Design review of the part built by this model. Coordinates are the model's own, in mm. Face numbers are marked on the shaded views. A direction names the side the tool comes from. Give positions to 0.01 mm unless a question says otherwise; leave off trailing zeros. Write each loop counter-clockwise with the first axis right and the second up, starting at its lowest first coordinate (ties: lowest second). Pieces come first, ordered by that corner, then holes. Notation, with made-up numbers: (-30, -37) -> (-11, -37) arc R3 cw to (-11, -33) -> close; hole circle Ø8 at (38.5, 11.5). An arc over 180 degrees is marked (long way). Write each question's results on one line, items separated by ' | '. Start each with the question number.
(1) Take a section at C-C (x = 117). State the section outline as (y, z) points.
(2) Take a section at D-D (x = 39). State the section outline as (y, z) points.
(3) For the marked faces 1 and 2, list the 3-axis set-ups (+Z, -Z, +X, -X, +Y, -Y) from which the entire face can be reached by the end or side of a thin tool; tool diameter is ignored.
(4) Take a section at A-A (x = -63). State the section outline as (y, z) points.
(5) Clearance check with flat-ended pins moving along their axes: pin 1 (5 mm diameter, centred on x = 9, y = 28.5, fed in from -Z); pin 2 (10 mm diameter, centred on y = 8.5, z = -33, fed in from +X); pin 3 (1.5 mm diameter, centred on y = 30, z = -1, fed in from +X); pin 4 (9 mm diameter, centred on x = 20.99, z = -20.99, fed in from +Y). State where each tip first meets the part, or that it passes through.
(6) Take a section at B-B (y = 2.5). Count the separate pieces of the cut face and the enclosed holes in it, plus the area to 3 significant figures.
(7) Mouldability with a two-part tool opening along Z and no side actions: class the marked faces 3, 4 and 5 as released by +Z, released by -Z, zero draft, split by the parting line, or undercut.
(8) To check wall thickness, follow probe 1 along Z at (x, y) = (-65, 11); probe 2 along Z at (x, y) = (-28, 6); probe 3 along Z at (x, y) = (16.5, 32). State the ranges of each line that lie inside material, in increasing order.
from build123d import *

# Parameters (mm, degrees)
BOSS_EXTRUDE3_DEPTH = 35
SKETCH1_8_R         = 4.99771167
SKETCH1_8_R_2       = 3.998169336
BOSS_EXTRUDE4_DEPTH = 5
CUT_EXTRUDE1_DEPTH  = 10
BOSS_EXTRUDE5_START = -3
SKETCH22_R          = 3
BOSS_EXTRUDE5_DEPTH = 3
SKETCH2_R           = 12
SKETCH2_R_2         = 9.5
BOSS_EXTRUDE6_DEPTH = 29
SKETCH23_R          = 3
SKETCH23_R_2        = 2.999999999
BOSS_EXTRUDE7_DEPTH = 4
SKETCH11_R          = 1.5
SKETCH11_R_2        = 11.25
CUT_EXTRUDE2_DEPTH  = 20
SKETCH24_R          = 4
SKETCH24_R_2        = 2.5
SKETCH24_R_3        = 3.5
SKETCH24_R_4        = 2.500018474
BOSS_EXTRUDE8_DEPTH = 30


with BuildPart() as part:
    # Sketch1 → Boss-Extrude3 (new body)
    with BuildSketch(Plane(origin=(0, 0, 0), x_dir=(1, 0, 0), z_dir=(0, 1, 0))):
        with BuildLine():
            Line((-86.695031893, 25.988113322), (-86.695031893, -25.991886678))
            Line((-86.695031893, -25.991886678), (-39.189227367, -25.991886678))
            ThreePointArc((-39.189227367, -25.991886678), (-7.506053104, -46.403541136), (28.985180603, -36.977564703))
            Line((28.985180603, -36.977564703), (84.985180603, -36.999994064))
            ThreePointArc((84.985180603, -36.999994064), (122.000000001, 2.968e-06), (84.985180603, 37))
            Line((84.985180603, 37), (28.985180603, 36.977570638))
            ThreePointArc((28.985180603, 36.977570638), (-7.510107434, 46.404944207), (-39.195031893, 25.988113322))
            Line((-39.195031893, 25.988113322), (-86.695031893, 25.988113322))
        make_face()
        with BuildLine():
            Line((-82.377665867, 22.997385422), (-82.377665867, -22.999994064))
            Line((-82.377665867, -22.999994064), (-37.526858967, -22.999994064))
            ThreePointArc((-37.526858967, -22.999994064), (-7.29337461, -43.394145047), (27.938898317, -33.977568435))
            Line((27.938898317, -33.977568435), (84.985180603, -34.00091317))
            ThreePointArc((84.985180603, -34.00091317), (119.000007777, -2.847e-06), (84.985180603, 34.000907476))
            Line((84.985180603, 34.000907476), (27.945855319, 33.977565588))
            ThreePointArc((27.945855319, 33.977565588), (-7.280719209, 43.388716375), (-37.507775535, 22.997385422))
            Line((-37.507775535, 22.997385422), (-82.377665867, 22.997385422))
        make_face(mode=Mode.SUBTRACT)
    extrude(amount=BOSS_EXTRUDE3_DEPTH)

    # Sketch22 → Boss-Extrude5 (add)
    with BuildSketch(Plane(origin=(0, 35, 0), x_dir=(1, 0, 0), z_dir=(0, 1, 0)).offset(BOSS_EXTRUDE5_START)):
        with BuildLine():
            ThreePointArc((126, -4), (130, 0), (126, 4))
            Line((126, 4), (121.783148639, 4))
            ThreePointArc((121.783148639, 4), (122.000000001, -1.7e-08), (121.783147994, -4))
            Line((121.783147994, -4), (126, -4))
        make_face()
        with Locations(Location((126, 0, 0), (0, 0, 270))):
            Circle(SKETCH22_R, mode=Mode.SUBTRACT)
    extrude(amount=BOSS_EXTRUDE5_DEPTH)


with BuildPart() as body_2:
    # Sketch1_8 → Boss-Extrude4 (new body)
    with BuildSketch(Plane(origin=(0, 0, 0), x_dir=(1, 0, 0), z_dir=(0, 1, 0))):
        with BuildLine():
            Line((-82.377665867, 22.997385422), (-82.377665867, -22.999994064))
            Line((-82.377665867, -22.999994064), (-37.526858967, -22.999994064))
            ThreePointArc((-37.526858967, -22.999994064), (-7.29337461, -43.394145047), (27.938898317, -33.977568435))
            Line((27.938898317, -33.977568435), (84.985180603, -34.00091317))
            ThreePointArc((84.985180603, -34.00091317), (119.000007777, -2.847e-06), (84.985180603, 34.000907476))
            Line((84.985180603, 34.000907476), (27.945855319, 33.977565588))
            ThreePointArc((27.945855319, 33.977565588), (-7.280719209, 43.388716375), (-37.507775535, 22.997385422))
            Line((-37.507775535, 22.997385422), (-82.377665867, 22.997385422))
        make_face()
        with Locations(Location((-20.990389016, 20.990389016, 0), (0, 0, 270))):
            Circle(SKETCH1_8_R, mode=Mode.SUBTRACT)
        with Locations(Location((20.990389016, 20.990389016, 0), (0, 0, 270))):
            Circle(SKETCH1_8_R, mode=Mode.SUBTRACT)
        with Locations(Location((20.990389016, -20.990389016, 0), (0, 0, 270))):
            Circle(SKETCH1_8_R, mode=Mode.SUBTRACT)
        with Locations(Location((-20.990389016, -20.990389016, 0), (0, 0, 270))):
            Circle(SKETCH1_8_R, mode=Mode.SUBTRACT)
        with Locations(Location((-21.98993135, 0, 0), (0, 0, 270))):
            Circle(SKETCH1_8_R_2, mode=Mode.SUBTRACT)
    extrude(amount=BOSS_EXTRUDE4_DEPTH)

    # Sketch3 → Cut-Extrude1 (cut)
    with BuildSketch(Plane(origin=(0, 5, 0), x_dir=(1, 0, 0), z_dir=(0, 1, 0))):
        with BuildLine():
            Line((-2.5, -13), (-2.5, -8))
            ThreePointArc((-2.5, -8), (0, -5.5), (2.5, -8))
            Line((2.5, -8), (2.5, -13))
            ThreePointArc((2.5, -13), (0, -15.5), (-2.5, -13))
        make_face()
        with BuildLine():
            Line((-2.5, 13), (-2.5, 8))
            ThreePointArc((-2.5, 8), (0, 5.5), (2.5, 8))
            Line((2.5, 8), (2.5, 13))
            ThreePointArc((2.5, 13), (0, 15.5), (-2.5, 13))
        make_face()
    extrude(amount=-CUT_EXTRUDE1_DEPTH, mode=Mode.SUBTRACT)


    add(part.part)  # Boss-Extrude6 merges part
    # Sketch2 → Boss-Extrude6 (add)
    # profile 1 of 4: a face of its own
    with BuildSketch(Plane(origin=(0, 5, 0), x_dir=(1, 0, 0), z_dir=(0, 1, 0))):
        with Locations(Location((-21, 21, 0), (0, 0, 90))):
            Circle(SKETCH2_R)
        with Locations(Location((-21, 21, 0), (0, 0, 90))):
            Circle(SKETCH2_R_2, mode=Mode.SUBTRACT)
    # profile 2 of 4: a face of its own
    with BuildSketch(Plane(origin=(0, 5, 0), x_dir=(1, 0, 0), z_dir=(0, 1, 0))):
        with Locations(Location((-21, -21, 0), (0, 0, 90))):
            Circle(SKETCH2_R)
        with Locations(Location((-21, -21, 0), (0, 0, 90))):
            Circle(SKETCH2_R_2, mode=Mode.SUBTRACT)
    # profile 3 of 4: a face of its own
    with BuildSketch(Plane(origin=(0, 5, 0), x_dir=(1, 0, 0), z_dir=(0, 1, 0))):
        with Locations(Location((21, -21, 0), (0, 0, 90))):
            Circle(SKETCH2_R)
        with Locations(Location((21, -21, 0), (0, 0, 90))):
            Circle(SKETCH2_R_2, mode=Mode.SUBTRACT)
    # profile 4 of 4: a face of its own
    with BuildSketch(Plane(origin=(0, 5, 0), x_dir=(1, 0, 0), z_dir=(0, 1, 0))):
        with Locations(Location((21, 21, 0), (0, 0, 90))):
            Circle(SKETCH2_R)
        with Locations(Location((21, 21, 0), (0, 0, 90))):
            Circle(SKETCH2_R_2, mode=Mode.SUBTRACT)
    extrude(amount=BOSS_EXTRUDE6_DEPTH)

    # Sketch23 → Boss-Extrude7 (add)
    # profile 1 of 2: a face of its own
    with BuildSketch(Plane(origin=(0, 35, 0), x_dir=(1, 0, 0), z_dir=(0, 1, 0))):
        with BuildLine():
            Line((77, -36.996795805), (77, -42))
            ThreePointArc((77, -42), (81.000000001, -46.000000001), (85.000000001, -42))
            Line((85.000000001, -42), (84.985180603, -36.999994064))
            Line((84.985180603, -36.999994064), (77, -36.996795805))
        make_face()
        with Locations(Location((81.000000001, -42, 0), (0, 0, 270))):
            Circle(SKETCH23_R, mode=Mode.SUBTRACT)
    # profile 2 of 2: a face of its own
    with BuildSketch(Plane(origin=(0, 35, 0), x_dir=(1, 0, 0), z_dir=(0, 1, 0))):
        with BuildLine():
            ThreePointArc((84.985180603, 37), (84.992590302, 37.000002226), (85.000000001, 37.000002968))
            Line((85.000000001, 37.000002968), (85.000000001, 42))
            ThreePointArc((85.000000001, 42), (81.000000001, 46.000000001), (77, 42))
            Line((77, 42), (77, 36.996801741))
            Line((77, 36.996801741), (84.985180603, 37))
        make_face()
        with Locations(Location((81.000000001, 42, 0), (0, 0, 270))):
            Circle(SKETCH23_R_2, mode=Mode.SUBTRACT)
    extrude(amount=-BOSS_EXTRUDE7_DEPTH)

    # Sketch11 → Cut-Extrude2 (cut)
    with BuildSketch(Plane(origin=(0, 5, 0), x_dir=(1, 0, 0), z_dir=(0, 1, 0))):
        with Locations(Location((-72.5, -15.5, 0), (0, 0, 270))):
            Circle(SKETCH11_R)
        with Locations(Location((-41.5, -15.5, 0), (0, 0, 270))):
            Circle(SKETCH11_R)
        with Locations(Location((-57, 0.008103654, 0), (0, 0, 270))):
            Circle(SKETCH11_R_2)
        with Locations(Location((-72.5, 15.5, 0), (0, 0, 270))):
            Circle(SKETCH11_R)
        with Locations(Location((-41.5, 15.5, 0), (0, 0, 270))):
            Circle(SKETCH11_R)
    extrude(amount=-CUT_EXTRUDE2_DEPTH, mode=Mode.SUBTRACT)

    # Sketch24 → Boss-Extrude8 (add)
    # profile 1 of 10: a face of its own
    with BuildSketch(Plane(origin=(0, 5, 0), x_dir=(1, 0, 0), z_dir=(0, 1, 0))):
        with Locations(Location((-78, -11, 0), (0, 0, 270))):
            Circle(SKETCH24_R)
        with Locations(Location((-78, -11, 0), (0, 0, 270))):
            Circle(SKETCH24_R_2, mode=Mode.SUBTRACT)
    # profile 2 of 10: a face of its own
    with BuildSketch(Plane(origin=(0, 5, 0), x_dir=(1, 0, 0), z_dir=(0, 1, 0))):
        with Locations(Location((-57, -18, 0), (0, 0, 270))):
            Circle(SKETCH24_R)
        with Locations(Location((-57, -18, 0), (0, 0, 270))):
            Circle(SKETCH24_R_2, mode=Mode.SUBTRACT)
    # profile 3 of 10: a face of its own
    with BuildSketch(Plane(origin=(0, 5, 0), x_dir=(1, 0, 0), z_dir=(0, 1, 0))):
        with Locations(Location((-78, 11, 0), (0, 0, 270))):
            Circle(SKETCH24_R)
        with Locations(Location((-78, 11, 0), (0, 0, 270))):
            Circle(SKETCH24_R_2, mode=Mode.SUBTRACT)
    # profile 4 of 10: a face of its own
    with BuildSketch(Plane(origin=(0, 5, 0), x_dir=(1, 0, 0), z_dir=(0, 1, 0))):
        with Locations(Location((-57, 18, 0), (0, 0, 270))):
            Circle(SKETCH24_R)
        with Locations(Location((-57, 18, 0), (0, 0, 270))):
            Circle(SKETCH24_R_2, mode=Mode.SUBTRACT)
    # profile 5 of 10: a face of its own
    with BuildSketch(Plane(origin=(0, 5, 0), x_dir=(1, 0, 0), z_dir=(0, 1, 0))):
        with Locations(Location((-9, -39, 0), (0, 0, 270))):
            Circle(SKETCH24_R_3)
        with Locations(Location((-9, -39, 0), (0, 0, 270))):
            Circle(SKETCH24_R_2, mode=Mode.SUBTRACT)
    # profile 6 of 10: a face of its own
    with BuildSketch(Plane(origin=(0, 5, 0), x_dir=(1, 0, 0), z_dir=(0, 1, 0))):
        with Locations(Location((9, -39, 0), (0, 0, 270))):
            Circle(SKETCH24_R_3)
        with Locations(Location((9, -39, 0), (0, 0, 270))):
            Circle(SKETCH24_R_2, mode=Mode.SUBTRACT)
    # profile 7 of 10: a face of its own
    with BuildSketch(Plane(origin=(0, 5, 0), x_dir=(1, 0, 0), z_dir=(0, 1, 0))):
        with Locations(Location((9, 39, 0), (0, 0, 270))):
            Circle(SKETCH24_R_3)
        with Locations(Location((9, 39, 0), (0, 0, 270))):
            Circle(SKETCH24_R_2, mode=Mode.SUBTRACT)
    # profile 8 of 10: a face of its own
    with BuildSketch(Plane(origin=(0, 5, 0), x_dir=(1, 0, 0), z_dir=(0, 1, 0))):
        with Locations(Location((-9, 39, 0), (0, 0, 270))):
            Circle(SKETCH24_R_3)
        with Locations(Location((-9, 39, 0), (0, 0, 270))):
            Circle(SKETCH24_R_2, mode=Mode.SUBTRACT)
    # profile 9 of 10: a face of its own
    with BuildSketch(Plane(origin=(0, 5, 0), x_dir=(1, 0, 0), z_dir=(0, 1, 0))):
        with BuildLine():
            ThreePointArc((44.829954146, 33.984474975), (42.233057283, 27.100010728), (49.000522442, 29.988113322))
            ThreePointArc((49.000522442, 29.988113322), (47.88749228, 32.756760132), (45.167819864, 33.984613237))
            Line((45.167819864, 33.984613237), (44.829954146, 33.984474975))
        make_face()
        with Locations(Location((45.000522442, 29.988113322, 0), (0, 0, 270))):
            Circle(SKETCH24_R_2, mode=Mode.SUBTRACT)
    # profile 10 of 10: a face of its own
    with BuildSketch(Plane(origin=(0, 5, 0), x_dir=(1, 0, 0), z_dir=(0, 1, 0))):
        with BuildLine():
            ThreePointArc((45.458576581, -33.984737916), (47.992614862, -32.669469565), (49.009082655, -30.001497662))
            ThreePointArc((49.009082655, -30.001497662), (42.332724858, -27.007262921), (44.537106836, -33.984360828))
            Line((44.537106836, -33.984360828), (45.458576581, -33.984737916))
        make_face()
        with Locations(Location((44.999471671, -30.001497662, 0), (0, 0, 270))):
            Circle(SKETCH24_R_4, mode=Mode.SUBTRACT)
    extrude(amount=BOSS_EXTRUDE8_DEPTH)


solid = body_2.part
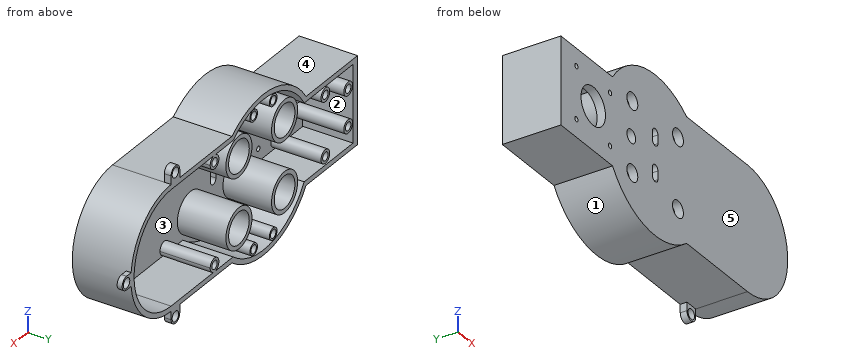
Report:
1) outline: (0, -18.57) -> (35, -18.57) -> (35, -11.49) -> (5, -11.49) -> (5, 11.49) -> (35, 11.49) -> (35, 18.57) -> (0, 18.57) -> close
2) outline: (0, -36.98) -> (35, -36.98) -> (35, -33.98) -> (5, -33.98) -> (5, 33.98) -> (35, 33.98) -> (35, 36.98) -> (0, 36.98) -> close
3) face 1: -Z, +Y, -Y | face 2: +Y
4) outline: (0, -25.99) -> (35, -25.99) -> (35, -23) -> (5, -23) -> (5, -9.52) -> (0, -9.52) -> close; (0, 9.51) -> (5, 9.51) -> (5, 23) -> (35, 23) -> (35, 25.99) -> (0, 25.99) -> close
5) pin 1: z = -46.55 | pin 2: x = 109.19 | pin 3: x = 122 | pin 4: through
6) separate pieces: 1 | enclosed holes: 12 | area: 13,600 mm2
7) face 3: undercut | face 4: released by +Z | face 5: zero draft
8) probe 1: -25.99 to -23, 23 to 25.99 | probe 2: -37.78 to -33.94, -30.75 to -27.42, -14.58 to -11.25, 11.25 to 14.58, 27.42 to 30.75, 33.96 to 37.77 | probe 3: -44 to -40.78, -32.12 to -29.37, -12.63 to -9.88, 9.88 to 12.63, 29.37 to 32.12, 40.78 to 44
